Geometry check sheet. Reference: the model listing, model coordinates, mm. Face numbers are marked on the shaded views. Coordinates: 2 decimals unless noted, no trailing zeros. Order: outer loops, then holes, each group sorted by start corner. A loop starts at its lowest first (then second) coordinate and runs counter-clockwise, first axis right, second up. Notation, with made-up numbers: (76, 85.25) - (102, 85.25) arc R28 cw to (102, 123.25) - close; hole circle Ø11 at (54.5, 44.25). An arc over 180 degrees is marked (long way). Use CSV: the item, a comma, the result in double quotes. Start each with the question number.
1) Sectioned sample at B-B, the plane z = 3.9. Record the cut outline in (x, y).
2) Thickness scan on probe 1 along X at (y, z) = (55, 3.05); probe 2 along X at (y, z) = (-30, 3.15); probe 3 along Y at (x, z) = (-13, 3.55). Record the ranges inside material, lowest first. Write a range as [from, to].
3) Depth check by flat-ended pin: P1, Ø2, axis at x = 55.5, y = 14, coming from the +Z side; P2, Ø1.5, axis at x = -1.5, z = 1, coming from the +Y side; P3, Ø0.6, axis at x = -21.5, z = 4.5, coming from the -Y side. Enter the tip coordinate at first touch or a pass-through.
4) Sectioned sample at C-C, the plane x = 12.5. Record the cut outline in (y, z).
5) Draft check along Y on the marked faces 1 and 2. Enter one of: released by +Y, released by -Y, zero draft, split by the parting line, or undercut.
6) Sectioned sample at D-D, the plane y = 11.5. Record the cut outline in (x, z), and give its area (3 significant figures).
7) Sectioned sample at A-A, the plane y = 66.5. Record the cut outline in (x, z).
from build123d import *

# Parameters (mm, degrees)
RESSALTO_EXTRUS_O1_DEPTH = 3
RESSALTO_EXTRUS_O2_DEPTH = 2


with BuildPart() as part:
    # Esboço1 → Ressalto-extrusão1 (new body)
    with BuildSketch(Plane.XY):
        with BuildLine():
            Line((-58, 35.5), (-58, 80.5))
            Line((-58, 80.5), (-82, 80.5))
            Line((-82, 80.5), (-82, -39.5))
            ThreePointArc((-82, -39.5), (-76.142135624, -53.642135624), (-62, -59.5))
            Line((-62, -59.5), (62, -59.5))
            ThreePointArc((62, -59.5), (76.142135624, -53.642135624), (82, -39.5))
            Line((82, -39.5), (82, 80.5))
            Line((82, 80.5), (58, 80.5))
            Line((58, 80.5), (58, 35.5))
            Line((58, 35.5), (9.5, 35.5))
            Line((9.5, 35.5), (9.5, 42.5))
            Line((9.5, 42.5), (-9.5, 42.5))
            Line((-9.5, 42.5), (-9.5, 35.5))
            Line((-9.5, 35.5), (-58, 35.5))
        make_face()
    extrude(amount=RESSALTO_EXTRUS_O1_DEPTH)

    # Esboço2 → Ressalto-extrusão2 (add)
    with BuildSketch(Plane.XY.offset(3)):
        with BuildLine():
            Line((-8.5, 34.5), (-59, 34.5))
            Line((-59, 34.5), (-59, 79.5))
            Line((-59, 79.5), (-81, 79.5))
            Line((-81, 79.5), (-81, -39.5))
            ThreePointArc((-81, -39.5), (-75.435028843, -52.935028843), (-62, -58.5))
            Line((-62, -58.5), (62, -58.5))
            ThreePointArc((62, -58.5), (75.435028843, -52.935028843), (81, -39.5))
            Line((81, -39.5), (81, 79.5))
            Line((81, 79.5), (59, 79.5))
            Line((59, 79.5), (59, 34.5))
            Line((59, 34.5), (8.5, 34.5))
            Line((8.5, 34.5), (8.5, 41.5))
            Line((8.5, 41.5), (-8.5, 41.5))
            Line((-8.5, 41.5), (-8.5, 34.5))
        make_face()
        with BuildLine():
            Line((-80, 78.5), (-80, -39.5))
            ThreePointArc((-80, -39.5), (-74.727922061, -52.227922061), (-62, -57.5))
            Line((-62, -57.5), (62, -57.5))
            ThreePointArc((62, -57.5), (74.727922061, -52.227922061), (80, -39.5))
            Line((80, -39.5), (80, 78.5))
            Line((80, 78.5), (60, 78.5))
            Line((60, 78.5), (60, 33.5))
            Line((60, 33.5), (7.5, 33.5))
            Line((7.5, 33.5), (7.5, 40.5))
            Line((7.5, 40.5), (-7.5, 40.5))
            Line((-7.5, 40.5), (-7.5, 33.5))
            Line((-7.5, 33.5), (-60, 33.5))
            Line((-60, 33.5), (-60, 78.5))
            Line((-60, 78.5), (-80, 78.5))
        make_face(mode=Mode.SUBTRACT)
    extrude(amount=RESSALTO_EXTRUS_O2_DEPTH)


solid = part.part
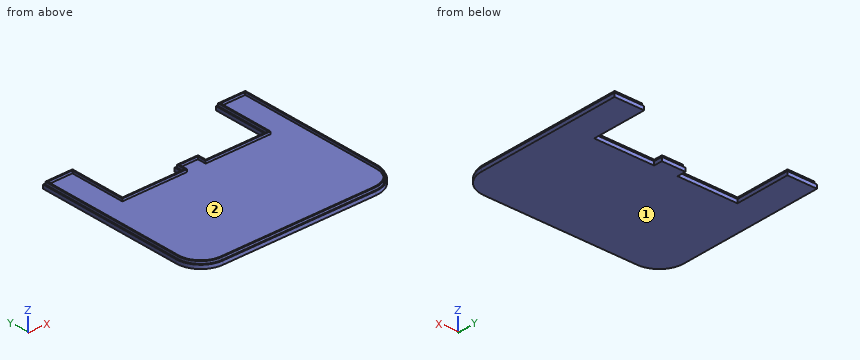
Evaluation:
1,outline,"(-81, -39.5) arc R19 ccw to (-62, -58.5) - (62, -58.5) arc R19 ccw to (81, -39.5) - (81, 79.5) - (59, 79.5) - (59, 34.5) - (8.5, 34.5) - (8.5, 41.5) - (-8.5, 41.5) - (-8.5, 34.5) - (-59, 34.5) - (-59, 79.5) - (-81, 79.5) - close; hole (-80, -39.5) arc R18 ccw to (-62, -57.5) - (62, -57.5) arc R18 ccw to (80, -39.5) - (80, 78.5) - (60, 78.5) - (60, 33.5) - (7.5, 33.5) - (7.5, 40.5) - (-7.5, 40.5) - (-7.5, 33.5) - (-60, 33.5) - (-60, 78.5) - (-80, 78.5) - close"
2,probe 1,"[-81, -80], [-60, -59], [59, 60], [80, 81]"
2,probe 2,"[-81, -80], [80, 81]"
2,probe 3,"[-58.5, -57.5], [33.5, 34.5]"
3,P1,"z = 3"
3,P2,"y = 42.5"
3,P3,"y = -58.5"
4,outline,"(-59.5, 0) - (35.5, 0) - (35.5, 3) - (34.5, 3) - (34.5, 5) - (33.5, 5) - (33.5, 3) - (-57.5, 3) - (-57.5, 5) - (-58.5, 5) - (-58.5, 3) - (-59.5, 3) - close"
5,face 1,"zero draft"
5,face 2,"undercut"
6,outline,"(-82, 0) - (82, 0) - (82, 3) - (81, 3) - (81, 5) - (80, 5) - (80, 3) - (-80, 3) - (-80, 5) - (-81, 5) - (-81, 3) - (-82, 3) - close"
6,area,"496 mm²"
7,outline,"(-82, 0) - (-58, 0) - (-58, 3) - (-59, 3) - (-59, 5) - (-60, 5) - (-60, 3) - (-80, 3) - (-80, 5) - (-81, 5) - (-81, 3) - (-82, 3) - close; (58, 0) - (82, 0) - (82, 3) - (81, 3) - (81, 5) - (80, 5) - (80, 3) - (60, 3) - (60, 5) - (59, 5) - (59, 3) - (58, 3) - close"
